Here's how the part is built. I have some questions about the finished solid (model axes, mm). A direction names the side the tool comes from. Give positions to 0.01 mm unless a question says otherwise; leave off trailing zeros. Order: outer loops, then holes, each group sorted by start corner. A loop starts at its lowest first (then second) coordinate and runs counter-clockwise, first axis right, second up. Notation, with made-up numbers: (-33, 10.5) -> (-15, 10.5) arc R16 ccw to (-15, 33.5) -> close; hole circle Ø10 at (62.5, 60.25). An arc over 180 degrees is marked (long way). Write each question's results on one line, items separated by ' | '. Start each with the question number.
Q1. Imagine slicing it at B-B, the plane z = 0.5. Please give me the cut outline in (x, y).
Q2. Thinking about a two-plate mould opening in X: for faces 3 (the face through (78.55, 7.93, 0.49)), 4 (the face through (74, 16, 1)), 5 (the face through (74.51, 8.07, 0.49)), 6 (the face through (150.5, 9.7, 0.8)), which applies, pulls with the +X half, pulls with the -X half, needs draft (parallel to the pull), parting line crosses it, or undercut?
Q3. I need wall thicknesses on line 1 along X through (y, z) = (5.5, 0.6); line 2 along Y through (x, z) = (21, 0.2); line 3 along Y through (x, z) = (84, 1.9). Which ranges of each line are inside material? Lowest first, please. Write a range as [from, to].
Q4. Imagine slicing it at C-C, the plane y = 9.25. Please give me the cut outline in (x, z).
Q5. Imagine slicing it at A-A, the plane x = 121. Please give me the cut outline in (y, z), then the cut area to 3 significant figures.
Q6. I'm going to push flat-ended pins straight in: pin 1 (1 mm diameter, centred on x = 71, y = 6, fed in from -Z); pin 2 (0.6 mm diameter, centred on y = 8, z = 1.5, fed in from +X); pin 3 (7 mm diameter, centred on x = 48, y = 6.5, fed in from +Z). Where does each tip first touch, or does it pass through?
Q7. For faces 1 (the face through (75, 15, 3)), 2 (the face through (75, 10, 1)), which set-ups out of +Z, -Z, +X, -X, +Y, -Y let a thin tool reach every point of the face, with its end or its side?
```python
from build123d import *

# Parameters (mm, degrees)
BOX020_W      = 30
BOX020_H      = 7
BOX020_DEPTH  = 10
BOX027_W      = 30
BOX027_H      = 7
BOX027_DEPTH  = 10
BOX028_W      = 30
BOX028_H      = 7
BOX028_DEPTH  = 10
BOX026_W      = 30
BOX026_H      = 7
BOX026_DEPTH  = 10
EXTRUDE_DEPTH = 4
BOX019_W      = 148.5
BOX019_H      = 14
BOX019_DEPTH  = 2
BOX014_W      = 150.5
BOX014_H      = 16
BOX014_DEPTH  = 3


with BuildPart() as cube020:
    # Box020 → Box020 (new body)
    with BuildSketch(Plane(origin=(6, 3.5, -3), x_dir=(1, 0, 0), z_dir=(0, 0, 1))):
        with Locations((15, 3.5)):
            Rectangle(BOX020_W, BOX020_H)
    extrude(amount=BOX020_DEPTH)


with BuildPart() as cube027:
    # Box027 → Box027 (new body)
    with BuildSketch(Plane(origin=(83, 3.5, -3), x_dir=(1, 0, 0), z_dir=(0, 0, 1))):
        with Locations((15, 3.5)):
            Rectangle(BOX027_W, BOX027_H)
    extrude(amount=BOX027_DEPTH)


with BuildPart() as cube028:
    # Box028 → Box028 (new body)
    with BuildSketch(Plane(origin=(118, 3.5, -3), x_dir=(1, 0, 0), z_dir=(0, 0, 1))):
        with Locations((15, 3.5)):
            Rectangle(BOX028_W, BOX028_H)
    extrude(amount=BOX028_DEPTH)


with BuildPart() as cube026:
    # Box026 → Box026 (new body)
    with BuildSketch(Plane(origin=(39, 3.5, -3), x_dir=(1, 0, 0), z_dir=(0, 0, 1))):
        with Locations((15, 3.5)):
            Rectangle(BOX026_W, BOX026_H)
    extrude(amount=BOX026_DEPTH)


with BuildPart() as extrude_body:
    # Sketch (on Face7 of Cut009) → Extrude (new body)
    with BuildSketch(Plane.XY.offset(1)):
        Polygon((76.5, 12), (72.459738, 2), (80.540262, 2), align=None)
    extrude(amount=EXTRUDE_DEPTH)


with BuildPart() as extrude_body_1:
    # Extrude placement: moved
    add(extrude_body.part.moved(Location((0, 1, -2.3))))


with BuildPart() as cube019:
    # Box019 → Box019 (new body)
    with BuildSketch(Plane(origin=(2, 0, 1), x_dir=(1, 0, 0), z_dir=(0, 0, 1))):
        with Locations((74.25, 7)):
            Rectangle(BOX019_W, BOX019_H)
    extrude(amount=BOX019_DEPTH)


with BuildPart() as obj1:
    # Box014 → Box014 (new body)
    with BuildSketch(Plane.XY):
        with Locations((75.25, 8)):
            Rectangle(BOX014_W, BOX014_H)
    extrude(amount=BOX014_DEPTH)

    # Cut009: cut Cube019
    add(cube019.part, mode=Mode.SUBTRACT)

    # Cut010: cut Extrude body
    add(extrude_body_1.part, mode=Mode.SUBTRACT)

    # Cut011: cut Cube026
    add(cube026.part, mode=Mode.SUBTRACT)

    # Cut012: cut Cube028
    add(cube028.part, mode=Mode.SUBTRACT)

    # Cut013: cut Cube027
    add(cube027.part, mode=Mode.SUBTRACT)

    # Cut014: cut Cube020
    add(cube020.part, mode=Mode.SUBTRACT)


solid = obj1.part
```
Geometry check:
1) outline: (0, 0) -> (150.5, 0) -> (150.5, 16) -> (0, 16) -> close; hole (6, 3.5) -> (36, 3.5) -> (36, 10.5) -> (6, 10.5) -> close; hole (39, 3.5) -> (69, 3.5) -> (69, 10.5) -> (39, 10.5) -> close; hole (72.46, 3) -> (80.54, 3) -> (76.5, 13) -> close; hole (83, 3.5) -> (113, 3.5) -> (113, 10.5) -> (83, 10.5) -> close; hole (118, 3.5) -> (148, 3.5) -> (148, 10.5) -> (118, 10.5) -> close
2) face 3: undercut | face 4: needs draft | face 5: undercut | face 6: pulls with the +X half
3) line 1: [0, 6], [36, 39], [69, 73.47], [79.53, 83], [113, 118], [148, 150.5] | line 2: [0, 3.5], [10.5, 16] | line 3: [14, 16]
4) outline: (0, 0) -> (6, 0) -> (6, 1) -> (2, 1) -> (2, 3) -> (0, 3) -> close; (36, 0) -> (39, 0) -> (39, 1) -> (36, 1) -> close; (69, 0) -> (74.98, 0) -> (74.98, 1) -> (69, 1) -> close; (78.02, 0) -> (83, 0) -> (83, 1) -> (78.02, 1) -> close; (113, 0) -> (118, 0) -> (118, 1) -> (113, 1) -> close; (148, 0) -> (150.5, 0) -> (150.5, 1) -> (148, 1) -> close
5) outline: (0, 0) -> (3.5, 0) -> (3.5, 1) -> (0, 1) -> close; (10.5, 0) -> (16, 0) -> (16, 3) -> (14, 3) -> (14, 1) -> (10.5, 1) -> close | area: 13.0 mm²
6) pin 1: z = 0 | pin 2: x = 2 | pin 3: z = 1
7) face 1: +Z, +X, -X, +Y, -Y | face 2: +Z, +X, -Y
